The figure shows three views and two pictorial views of one solid part (mm, origin at its lowest corner). Answer the questions. Round coordinates to 2 decimals unless told otherwise and drop trailing zeros. Write each loop counter-clockwise with the first axis right and the second up, starting at its lowest first coordinate (ties: lowest second). Pieces come first, ordered by that corner, then holes. Notation, with made-up numbers: M 59,-24 L 64,-24 A31 ccw 64,11 Z; hole C 64.5,6.5 d3. An arc over 180 degrees is marked long. One line per item, written item: value. Start each with the question number.
Q1. Consider probe 1 along Y at (x, z) = (73.5, 3) (1 decimal); probe 2 along Z at (x, y) = (47, 18.75); probe 3 along Y at (x, z) = (6, 5). Determine where each line is inside the solid, lowest interval first.
Q2. The mould has two halves that part along X. Classify the marked faces 1 and 2: released by +X, released by -X, zero draft, split by the parting line, or undercut.
Q3. Find section C-C (z = 4.75). Write down the section's boundary in (x, y), and give its area (3 significant figures).
Q4. Find section B-B (y = 18.75). Write down the section's boundary in (x, z), and give its area (3 significant figures).
Q5. Find section A-A (x = 29.5). Write down the section's boundary in (y, z).
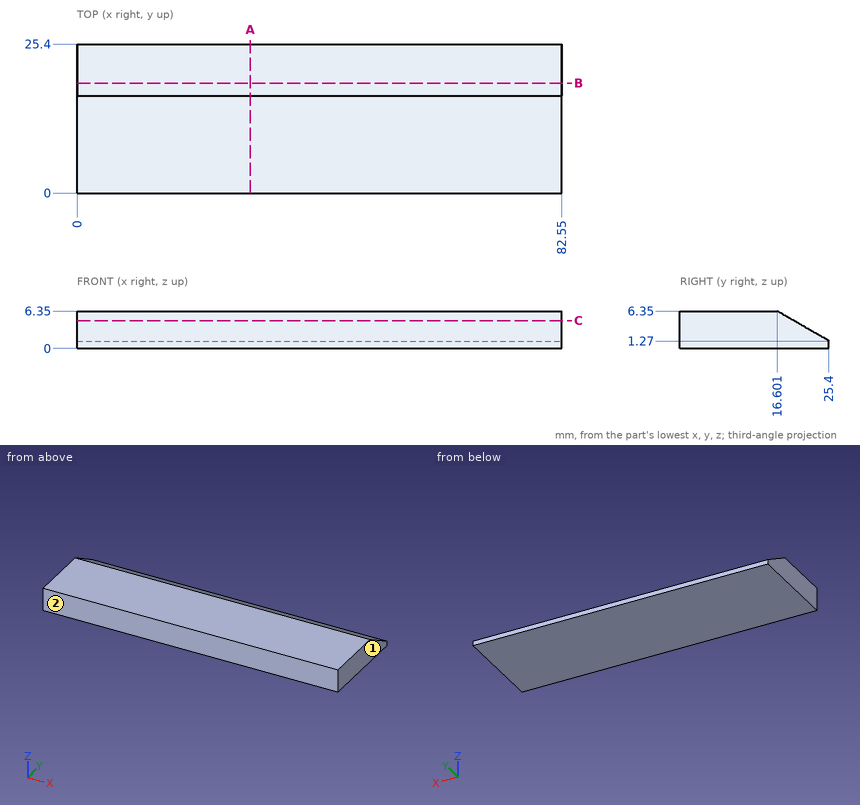
The answers:
1. probe 1: 0 to 22.4
1. probe 2: 0 to 5.11
1. probe 3: 0 to 18.94
2. face 1: released by +X
2. face 2: zero draft
3. outline: M 0,0 L 82.55,0 L 82.55,19.37 L 0,19.37 Z
3. area: 1,600 mm2
4. outline: M 0,0 L 82.55,0 L 82.55,5.11 L 0,5.11 Z
4. area: 422 mm2
5. outline: M 0,0 L 25.4,0 L 25.4,1.27 L 16.6,6.35 L 0,6.35 Z
